```python
from build123d import *

# Parameters (mm, degrees)
SKETCH1_R           = 28.4
SKETCH1_R_2         = 5
SKETCH1_R_3         = 3
BOSS_EXTRUDE3_DEPTH = 6
SKETCH5_R           = 12
SKETCH5_R_2         = 5
BOSS_EXTRUDE4_DEPTH = 20.4


with BuildPart() as part:
    # Sketch1 → Boss-Extrude3 (new body)
    with BuildSketch(Plane(origin=(0, 0, 0), x_dir=(1, 0, 0), z_dir=(0, 1, 0))):
        Circle(SKETCH1_R)
        Circle(SKETCH1_R_2, mode=Mode.SUBTRACT)
        with Locations((0, 23.75)):
            Circle(SKETCH1_R_3, mode=Mode.SUBTRACT)
        with Locations((20.56810334, 11.875)):
            Circle(SKETCH1_R_3, mode=Mode.SUBTRACT)
        with Locations((20.56810334, -11.875)):
            Circle(SKETCH1_R_3, mode=Mode.SUBTRACT)
        with Locations((0, -23.75)):
            Circle(SKETCH1_R_3, mode=Mode.SUBTRACT)
        with Locations((-20.56810334, -11.875)):
            Circle(SKETCH1_R_3, mode=Mode.SUBTRACT)
        with Locations((-20.56810334, 11.875)):
            Circle(SKETCH1_R_3, mode=Mode.SUBTRACT)
    extrude(amount=BOSS_EXTRUDE3_DEPTH)

    # Sketch5 → Boss-Extrude4 (add)
    with BuildSketch(Plane(origin=(0, 6, 0), x_dir=(1, 0, 0), z_dir=(0, 1, 0))):
        Circle(SKETCH5_R)
        Circle(SKETCH5_R_2, mode=Mode.SUBTRACT)
    extrude(amount=BOSS_EXTRUDE4_DEPTH)


solid = part.part
```
Design review of the part built by this model. Coordinates are the model's own, in mm. A direction names the side the tool comes from. Coordinates: 2 decimals unless noted, no trailing zeros. Order: outer loops, then holes, each group sorted by start corner. A loop starts at its lowest first (then second) coordinate and runs counter-clockwise, first axis right, second up. Notation, with made-up numbers: M 38.25,71.25 L 42.25,71.25 A12 ccw 42.25,84.25 Z; hole C -29,-28.5 d1. An arc over 180 degrees is marked long. Answer as a JSON object with one key per item and string values. Group by question number.
1) For pin 1 (2 mm diameter, centred on y = 18.5, z = -5, fed in from -X); pin 2 (7 mm diameter, centred on x = 20.57, z = -11.88, fed in from +Y); pin 3 (1.5 mm diameter, centred on x = -10.5, y = 7, fed in from +Z), all flat-tipped, find the tip position at first contact; note any pin that passes through.
2) Wall thickness on L1, parallel to Z at x = 0, y = 2.55; L2, parallel to Z at x = -18, y = 5; L3, parallel to X at y = 5, z = -14.5: over which ranges is each line inside the solid? List them lowest first.
3) Add section D-D, the plane y = 12.5. Write out the cut boundary in (x, z).
4) Add section C-C, the plane x = 18.5. Write out the cut boundary in (y, z), then the cut area to 3 significant figures.
5) Add section B-B, the plane x = 0. Write out the cut boundary in (y, z).
6) Tool access review of faces 1 (the cylindrical face through (-11.99, 16.06, -0.53)), 2 (the cylindrical face through (-0.65, 2.96, 26.68)): name each direction out of +Z, -Z, +X, -X, +Y, -Y from which nothing blocks a thin tool from reaching the whole face with its end or side.
7) Add section A-A, the plane z = 0. Write out the cut boundary in (x, y), then the cut area to 3 significant figures.
8) Mouldability with a two-part tool opening along Z and no side actions: class faces 3 (the cylindrical face through (-3.697, 2.958, -28.158)), 4 (the flat face through (12.2, 6, -0.4)), 5 (the cylindrical face through (23.34, 2.96, -10.73)) as pulls with the +Z half, pulls with the -Z half, needs draft (parallel to the pull), parting line crosses it, or undercut.
Computed values:
{
 "1": {"pin 1": "stops at x = -11.31", "pin 2": "stops at y = 6", "pin 3": "stops at z = 7"},
 "2": {"L1": "z = -28.4 to -26.75, -20.75 to -5, 5 to 20.75, 26.75 to 28.4", "L2": "z = -21.97 to -13.43, -10.32 to 10.32, 13.43 to 21.97", "L3": "x = -24.42 to -22.02, -19.12 to 19.12, 22.02 to 24.42"},
 "3": {"outline": "C 0,0 d24; hole C 0,0 d10"},
 "4": {"outline": "M 0,-21.55 L 6,-21.55 L 6,-14.05 L 0,-14.05 Z; M 0,-9.7 L 6,-9.7 L 6,9.7 L 0,9.7 Z; M 0,14.05 L 6,14.05 L 6,21.55 L 0,21.55 Z", "area": "206 mm^2"},
 "5": {"outline": "M 0,-28.4 L 6,-28.4 L 6,-26.75 L 0,-26.75 Z; M 0,-20.75 L 6,-20.75 L 6,-12 L 26.4,-12 L 26.4,-5 L 0,-5 Z; M 0,5 L 26.4,5 L 26.4,12 L 6,12 L 6,20.75 L 0,20.75 Z; M 0,26.75 L 6,26.75 L 6,28.4 L 0,28.4 Z"},
 "6": {"face 1": "+Y", "face 2": "+Y, -Y"},
 "7": {"outline": "M -28.4,0 L -5,0 L -5,26.4 L -12,26.4 L -12,6 L -28.4,6 Z; M 5,0 L 28.4,0 L 28.4,6 L 12,6 L 12,26.4 L 5,26.4 Z", "area": "566 mm^2"},
 "8": {"face 3": "parting line crosses it", "face 4": "needs draft", "face 5": "undercut"}
}
